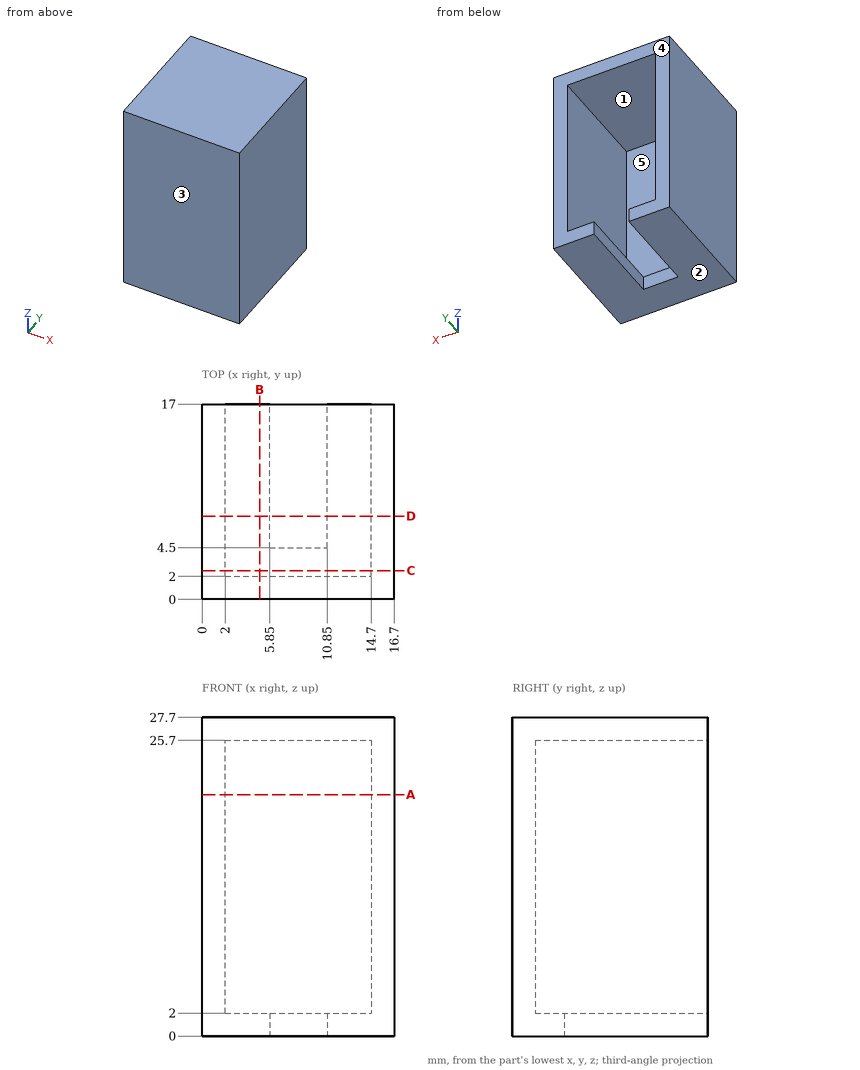
The drawing under review shows one solid part. Ordinate dimensions are in mm from its lowest x, y, z. A direction names the side the tool comes from. Round coordinates to 2 decimals unless told otherwise and drop trailing zeros. Order: outer loops, then holes, each group sorted by start corner. A loop starts at its lowest first (then second) coordinate and runs counter-clockwise, first axis right, second up. Notation, with made-up numbers: (-37, 88) - (-11, 88) arc R28 cw to (-11, 124) - close; hole circle Ø8 at (-39, 37.5). An arc over 180 degrees is marked (long way). Return JSON: item names as keys, results as strings.
Q1. Consider section C-C on y = 2.5. Write out the cut boundary in (x, z).
Computed values:
{"outline": "(0, 0) - (16.7, 0) - (16.7, 27.7) - (0, 27.7) - close; hole (2, 2) - (14.7, 2) - (14.7, 25.7) - (2, 25.7) - close"}
Q2. Machinability: for the marked faces 4 and 5, which of the approach directions +Z, -Z, +X, -X, +Y, -Y give a long, thin tool a straight path to every point of the face, cutting with its end or side? Answer none if there is none.
Computed values:
{"face 4": "+Z, -Z, +X, -X, +Y", "face 5": "+Y"}
Q3. Consider section A-A on z = 21. Write out the cut boundary in (x, y).
Computed values:
{"outline": "(0, 0) - (16.7, 0) - (16.7, 17) - (14.7, 17) - (14.7, 2) - (2, 2) - (2, 17) - (0, 17) - close"}
Q4. The part is to be moulded in two halves that separate along Z. For the marked faces 1, 2 and 3, say which applies: pulls with the +Z half, pulls with the -Z half, needs draft (parallel to the pull), parting line crosses it, or undercut.
Computed values:
{"face 1": "undercut", "face 2": "pulls with the -Z half", "face 3": "needs draft"}
Q5. Consider section B-B on x = 5. Write out the cut boundary in (y, z).
Computed values:
{"outline": "(0, 0) - (17, 0) - (17, 2) - (2, 2) - (2, 25.7) - (17, 25.7) - (17, 27.7) - (0, 27.7) - close"}
Q6. Wall thickness on L1, parallel to X at y = 10.5, z = 18.75; L2, parallel to Z at x = 13.75, y = 5; L3, parallel to Z at x = 8.5, y = 7.5: over which ranges is each line inside the solid? List them lowest first. Write a range as [from, to].
Computed values:
{"L1": "x = [0, 2], [14.7, 16.7]", "L2": "z = [0, 2], [25.7, 27.7]", "L3": "z = [25.7, 27.7]"}
Q7. For pin 1 Ø1.6 at (x, z) = (9.5, 1) entering from +Y; pin 2 Ø1 at (x, z) = (12.5, 11) entering from -Y; pin 3 Ø4 at (x, z) = (8.5, 19.5) entering from +Y, all flat-tipped, find the tip position at first contact; note any pin that passes through.
Computed values:
{"pin 1": "stops at y = 4.5", "pin 2": "stops at y = 0", "pin 3": "stops at y = 2"}
Q8. Consider section D-D on y = 7.25. Write out the cut boundary in (x, z).
Computed values:
{"outline": "(0, 0) - (5.85, 0) - (5.85, 2) - (2, 2) - (2, 25.7) - (14.7, 25.7) - (14.7, 2) - (10.85, 2) - (10.85, 0) - (16.7, 0) - (16.7, 27.7) - (0, 27.7) - close"}
